The figure shows three views and two pictorial views of one solid part (mm, origin at its lowest corner). Answer the questions. A direction names the side the tool comes from. Coordinates: 2 decimals unless noted, no trailing zeros. Write each loop counter-clockwise with the first axis right and the second up, starting at its lowest first coordinate (ties: lowest second). Pieces come first, ordered by that corner, then holes. Notation, with made-up numbers: M 55,-27.5 L 68,-27.5 A23 cw 68,0.5 Z; hole C -11,-36 d11. An arc over 180 degrees is marked long. Answer as CSV lines item,"result".
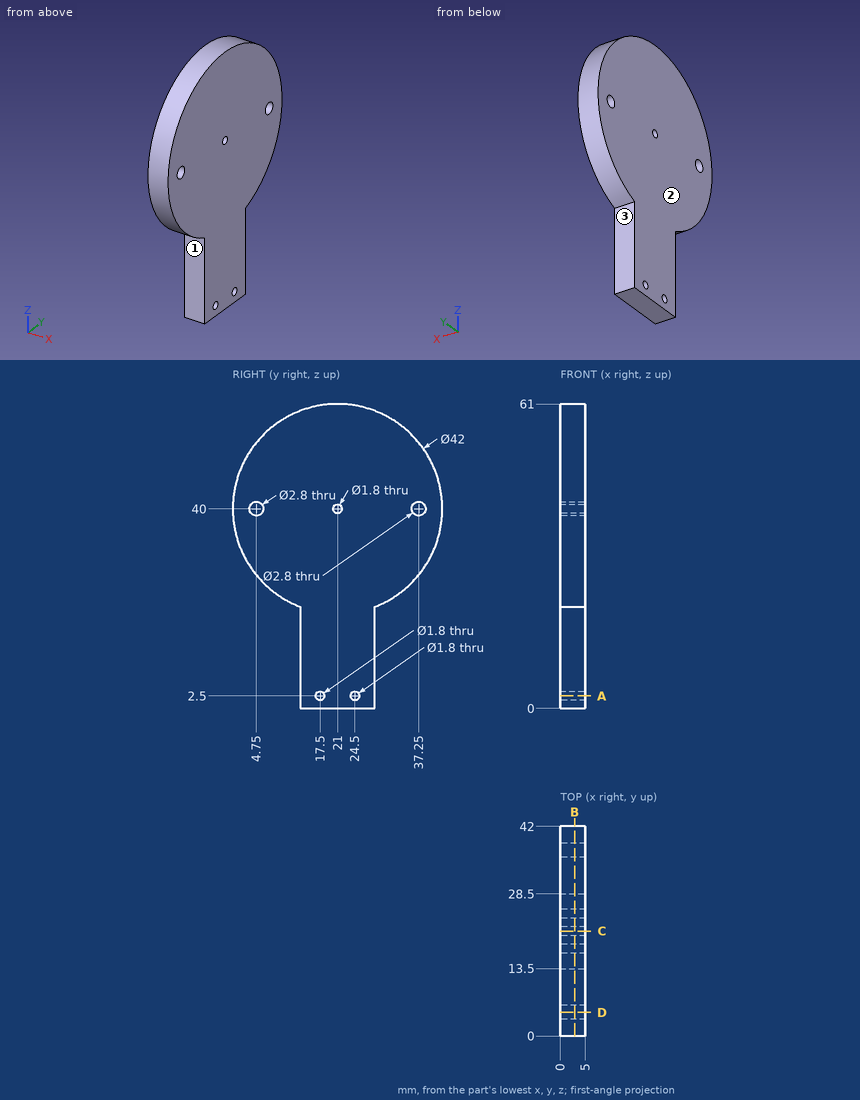
Q1. Flat-ended cylindrical pins translate along their axes: pin 1 Ø1 at (x, y) = (1.5, 13.5) entering from +Z; pin 2 Ø1.5 at (x, z) = (2, 19.5) entering from -Y; pin 3 Ø1 at (x, y) = (3, 30) entering from +Z. Find the tip coordinate at first contact, or state that the pin passes through.
Output:
pin 1,"z = 59.8"
pin 2,"y = 13.5"
pin 3,"z = 59.2"
Q2. Find section A-A (z = 2.5). Give the vertices of the cut face in (x, y).
Output:
outline,"M 0,13.5 L 5,13.5 L 5,16.6 L 0,16.6 Z; M 0,18.4 L 5,18.4 L 5,23.6 L 0,23.6 Z; M 0,25.4 L 5,25.4 L 5,28.5 L 0,28.5 Z"
Q3. Find section C-C (y = 21). Give the vertices of the cut face in (x, z).
Output:
outline,"M 0,0 L 5,0 L 5,39.1 L 0,39.1 Z; M 0,40.9 L 5,40.9 L 5,61 L 0,61 Z"
Q4. Find section B-B (x = 2.85). Give the vertices of the cut face in (y, z).
Output:
outline,"M 13.5,0 L 28.5,0 L 28.5,20.38 A21 ccw long 13.5,20.38 Z; hole C 4.75,40 d2.8; hole C 17.5,2.5 d1.8; hole C 21,40 d1.8; hole C 24.5,2.5 d1.8; hole C 37.25,40 d2.8"
Q5. For the marked faces 1, 2 and 3, determine the directions among +Z, -Z, +X, -X, +Y, -Y from which every point of the face is accessible in a straight line to the end or side of a thin tool.
Output:
face 1,"-Z, +X, -X, -Y"
face 2,"+Z, -Z, -X, +Y, -Y"
face 3,"-Z, +X, -X, +Y"
Q6. Straight lines are drawn through the part: line 1 (Y direction, x = 3.35, z = 40); line 2 (Y direction, x = 3, z = 4.5); line 3 (Z direction, x = 3.5, y = 4). For each, find the intervals that lie inside material, in ascending order.
Output:
line 1,"0 to 3.35, 6.15 to 20.1, 21.9 to 35.85, 38.65 to 42"
line 2,"13.5 to 28.5"
line 3,"27.67 to 38.82, 41.18 to 52.33"
Q7. Find section D-D (y = 4.75). Give the vertices of the cut face in (x, z), and give its area (3 significant figures).
Output:
outline,"M 0,26.7 L 5,26.7 L 5,38.6 L 0,38.6 Z; M 0,41.4 L 5,41.4 L 5,53.3 L 0,53.3 Z"
area,"119 mm2"
